Geometry: final body of the model. Coordinates: model frame, mm. Give positions to 0.01 mm unless a question says otherwise; leave off trailing zeros. Loops run counter-clockwise (first coordinate to the right, second up) from the corner with the lowest first, then second, coordinate; pieces in that order, holes last.
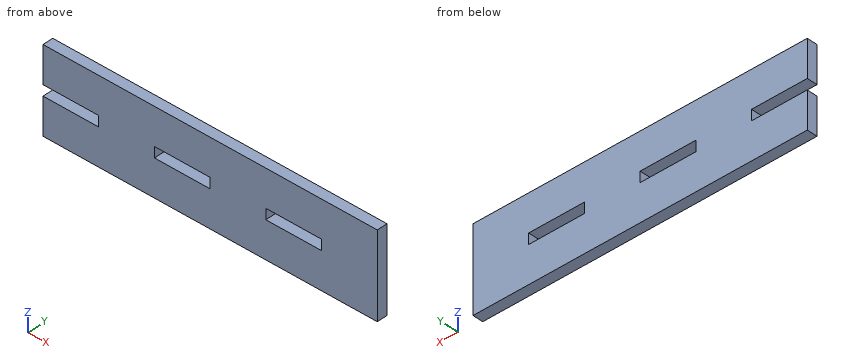
from build123d import *

# Parameters (mm, degrees)
SKETCH1_W           = 25.4
SKETCH1_H           = 4.7625
BOSS_EXTRUDE1_DEPTH = 4.7625


with BuildPart() as part:
    # Sketch1 → Boss-Extrude1 (new body)
    with BuildSketch(Plane(origin=(0, 0, 0), x_dir=(1, 0, 0), z_dir=(0, 1, 0))):
        Polygon((-76.2, 19.05), (-76.2, 2.38125), (-50.8, 2.38125), (-50.8, -2.38125), (-76.2, -2.38125), (-76.2, -19.05), (76.2, -19.05), (76.2, 19.05), align=None)
        with Locations((-12.7, 0)):
            Rectangle(SKETCH1_W, SKETCH1_H, mode=Mode.SUBTRACT)
        with Locations((38.1, 0)):
            Rectangle(SKETCH1_W, SKETCH1_H, mode=Mode.SUBTRACT)
    extrude(amount=BOSS_EXTRUDE1_DEPTH)


solid = part.part
Item 1: Section query B-B on y = 2.2. Return loops of the section in (x, z), plus the area to 3 significant figures.
Values follow:
outline: (-76.2, -19.05) - (76.2, -19.05) - (76.2, 19.05) - (-76.2, 19.05) - (-76.2, 2.38) - (-50.8, 2.38) - (-50.8, -2.38) - (-76.2, -2.38) - close; hole (-25.4, -2.38) - (0, -2.38) - (0, 2.38) - (-25.4, 2.38) - close; hole (25.4, -2.38) - (50.8, -2.38) - (50.8, 2.38) - (25.4, 2.38) - close
area: 5,440 mm2
Item 2: Section query A-A on x = 49.5. Return loops of the section in (y, z), plus the area to 3 significant figures.
Values follow:
outline: (0, -19.05) - (4.76, -19.05) - (4.76, -2.38) - (0, -2.38) - close; (0, 2.38) - (4.76, 2.38) - (4.76, 19.05) - (0, 19.05) - close
area: 159 mm2
Item 3: Ray query, probe 1 along X at (y, z) = (1.8, 2); probe 2 along Z at (x, y) = (-65, 4.1). Return the intervals inside material, ascending.
Values follow:
probe 1: x = -50.8 to -25.4, 0 to 25.4, 50.8 to 76.2
probe 2: z = -19.05 to -2.38, 2.38 to 19.05
Item 4: Pin query (flat end, axial travel): pin 1 (2.5 mm diameter, centred on y = 3.5, z = 0.5, fed in from -X). Return the tip coordinate at first contact, or that it passes through.
Values follow:
pin 1: stops at x = -50.8
